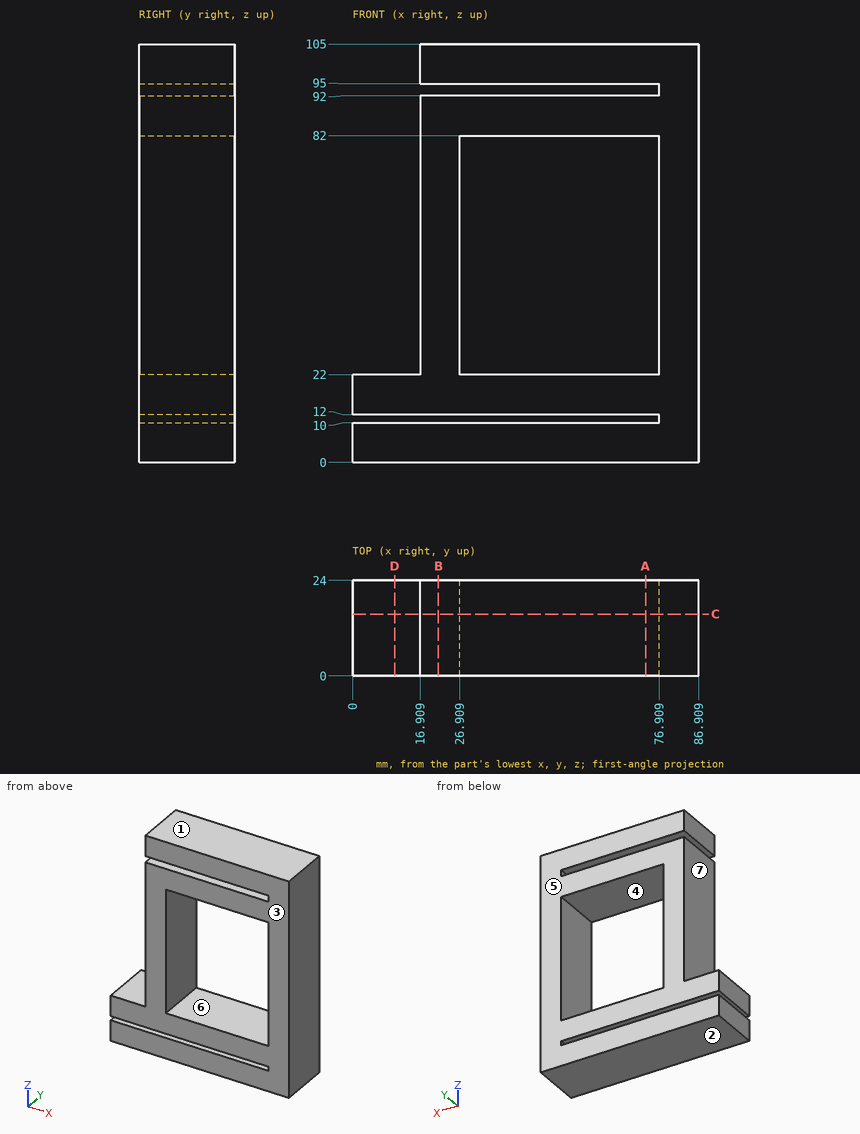
Source: three-view drawing plus pictorial views. Frame: mm from the lowest corner of the part. A direction names the side the tool comes from. Give positions to 0.01 mm unless a question says otherwise; leave off trailing zeros. Write each loop counter-clockwise with the first axis right and the second up, starting at its lowest first coordinate (ties: lowest second). Pieces come first, ordered by that corner, then holes. Notation, with made-up numbers: M -38,66.25 L 18,66.25 A21 ccw 18,98.25 Z; hole C 69.5,32 d7. An arc over 180 degrees is marked long. Use one line per item in the form item = value.
1. Cut plane D-D on x = 10.5. Return loops of the section in (y, z).
Outcome:
outline = M 0,0 L 24,0 L 24,10 L 0,10 Z; M 0,12 L 24,12 L 24,22 L 0,22 Z
2. Ray query, L1, parallel to Z at x = 44, y = 6; L2, parallel to Z at x = 9, y = 14.5; L3, parallel to X at y = 16.5, z = 22.5. Return the intervals inside material, ascending.
Outcome:
L1 = 0 to 10, 12 to 22, 82 to 92, 95 to 105
L2 = 0 to 10, 12 to 22
L3 = 16.91 to 26.91, 76.91 to 86.91
3. Cut plane C-C on y = 15.5. Return loops of the section in (x, z), and give its area (3 significant figures).
Outcome:
outline = M 0,0 L 86.91,0 L 86.91,105 L 16.91,105 L 16.91,95 L 76.91,95 L 76.91,92 L 16.91,92 L 16.91,22 L 0,22 L 0,12 L 76.91,12 L 76.91,10 L 0,10 Z; hole M 26.91,22 L 76.91,22 L 76.91,82 L 26.91,82 Z
area = 4,390 mm²
4. Cut plane A-A on x = 73.5. Return loops of the section in (y, z), and give its area (3 significant figures).
Outcome:
outline = M 0,0 L 24,0 L 24,10 L 0,10 Z; M 0,12 L 24,12 L 24,22 L 0,22 Z; M 0,82 L 24,82 L 24,92 L 0,92 Z; M 0,95 L 24,95 L 24,105 L 0,105 Z
area = 960 mm²
5. Mould query, pull axis Z, two halves, no side actions, for the marked faces 1, 2, 3 and 4. Classes: released by +Z, released by -Z, zero draft, split by the parting line, or undercut.
Outcome:
face_1 = released by +Z
face_2 = released by -Z
face_3 = zero draft
face_4 = undercut
6. Reachability of the marked faces 5, 6 and 7 from +Z, -Z, +X, -X, +Y, -Y: full face, straight path, thin tool, end or side. Return the list, or none.
Outcome:
face_5 = +Z, -Z, +X, -X, +Y
face_6 = +Y, -Y
face_7 = +Z, -X, +Y, -Y
7. Cut plane B-B on x = 21.5. Return loops of the section in (y, z).
Outcome:
outline = M 0,0 L 24,0 L 24,10 L 0,10 Z; M 0,12 L 24,12 L 24,92 L 0,92 Z; M 0,95 L 24,95 L 24,105 L 0,105 Z
8. First-contact query: P1, Ø5, axis at y = 6.5, z = 101.5, coming from the -X side; P2, Ø10, axis at x = 32.5, z = 57, coming from the -Y side; P3, Ø1.5, axis at y = 10, z = 93.5, coming from the -X side. Flat tips, straight axial feed; report the tip coordinate or a pass-through.
Outcome:
P1 = 16.91
P2 = through
P3 = 76.91
